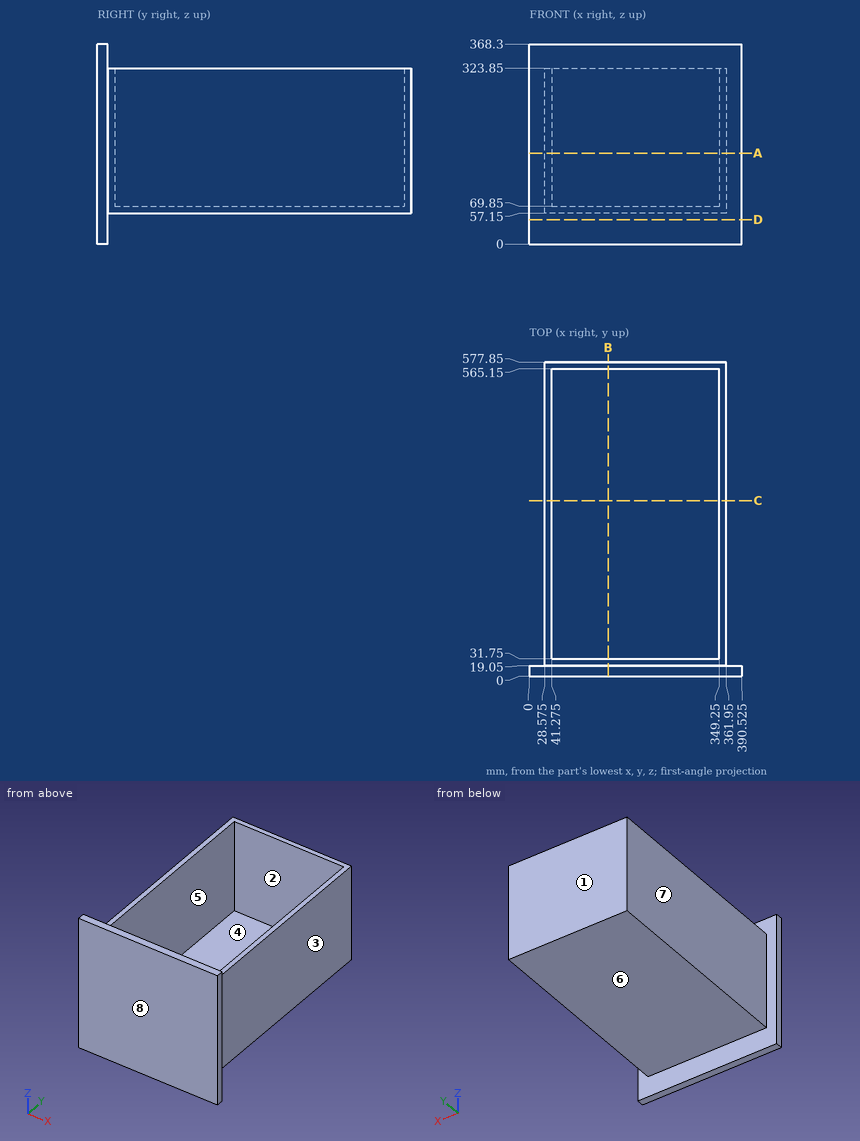
Input: dimensioned drawing with shaded views. Units: mm. Origin: part minimum x, y, z. A direction names the side the tool comes from. Round coordinates to 2 decimals unless told otherwise and drop trailing zeros. Order: outer loops, then holes, each group sorted by start corner. A loop starts at its lowest first (then second) coordinate and runs counter-clockwise, first axis right, second up. Notation, with made-up numbers: (-17.75, 13.5) - (37.25, 13.5) arc R9 cw to (37.25, 26.5) - close; hole circle Ø3 at (52, -7.5). An arc over 180 degrees is marked (long way). Answer as a JSON object with one key per item and string values. Group by question number.
(1) Reachability of the marked faces 5, 6, 7 and 8 from +Z, -Z, +X, -X, +Y, -Y: full face, straight path, thin tool, end or side. Return the list, or none.
(2) Draft query along Y for the marked faces 1, 2, 3 and 4. Return one class per face: released by +Y, released by -Y, zero draft, split by the parting line, or undercut.
(3) Cut plane D-D (z = 45). Return loops of the section in (x, y) (3 decimals).
(4) Cut plane C-C (y = 323). Return loops of the section in (x, z) (3 decimals).
(5) Cut plane A-A (z = 167.5). Return loops of the section in (x, y) (3 decimals).
(6) Cut plane B-B (x = 145). Return loops of the section in (y, z), then the cut area to 3 significant figures.
(7) Pin query (flat end, axial travel): P1, Ø5, axis at y = 71, z = 283.5, coming from the +X side; P2, Ø5, axis at x = 299.5, y = 356, coming from the -Z side; P3, Ø12, axis at x = 228.5, y = 416.5, coming from the +Z side. Return the tip coordinate at first contact, or that it passes through.
(8) Material intervals for probe 1 along X at (y, z) = (550, 92) (3 decimals); probe 2 along Y at (x, z) = (175, 76); probe 3 along Z at (x, y) = (201, 98), sorted ascending. Write a range as from..to.
Here are the results:
{
 "1": {"face 5": "+Z", "face 6": "-Z, +X, -X, +Y", "face 7": "+Z, -Z, -X, +Y", "face 8": "+Z, -Z, +X, -X, -Y"},
 "2": {"face 1": "released by +Y", "face 2": "undercut", "face 3": "zero draft", "face 4": "undercut"},
 "3": {"outline": "(0, 0) - (390.525, 0) - (390.525, 19.05) - (0, 19.05) - close"},
 "4": {"outline": "(28.575, 57.15) - (361.95, 57.15) - (361.95, 323.85) - (349.25, 323.85) - (349.25, 69.85) - (41.275, 69.85) - (41.275, 323.85) - (28.575, 323.85) - close"},
 "5": {"outline": "(0, 0) - (390.525, 0) - (390.525, 19.05) - (361.95, 19.05) - (361.95, 577.85) - (28.575, 577.85) - (28.575, 19.05) - (0, 19.05) - close; hole (41.275, 31.75) - (349.25, 31.75) - (349.25, 565.15) - (41.275, 565.15) - close"},
 "6": {"outline": "(0, 0) - (19.05, 0) - (19.05, 57.15) - (577.85, 57.15) - (577.85, 323.85) - (565.15, 323.85) - (565.15, 69.85) - (31.75, 69.85) - (31.75, 323.85) - (19.05, 323.85) - (19.05, 368.3) - (0, 368.3) - close", "area": "20,600 mm^2"},
 "7": {"P1": "stops at x = 361.95", "P2": "stops at z = 57.15", "P3": "stops at z = 69.85"},
 "8": {"probe 1": "x = 28.575..41.275, 349.25..361.95", "probe 2": "y = 0..31.75, 565.15..577.85", "probe 3": "z = 57.15..69.85"}
}
